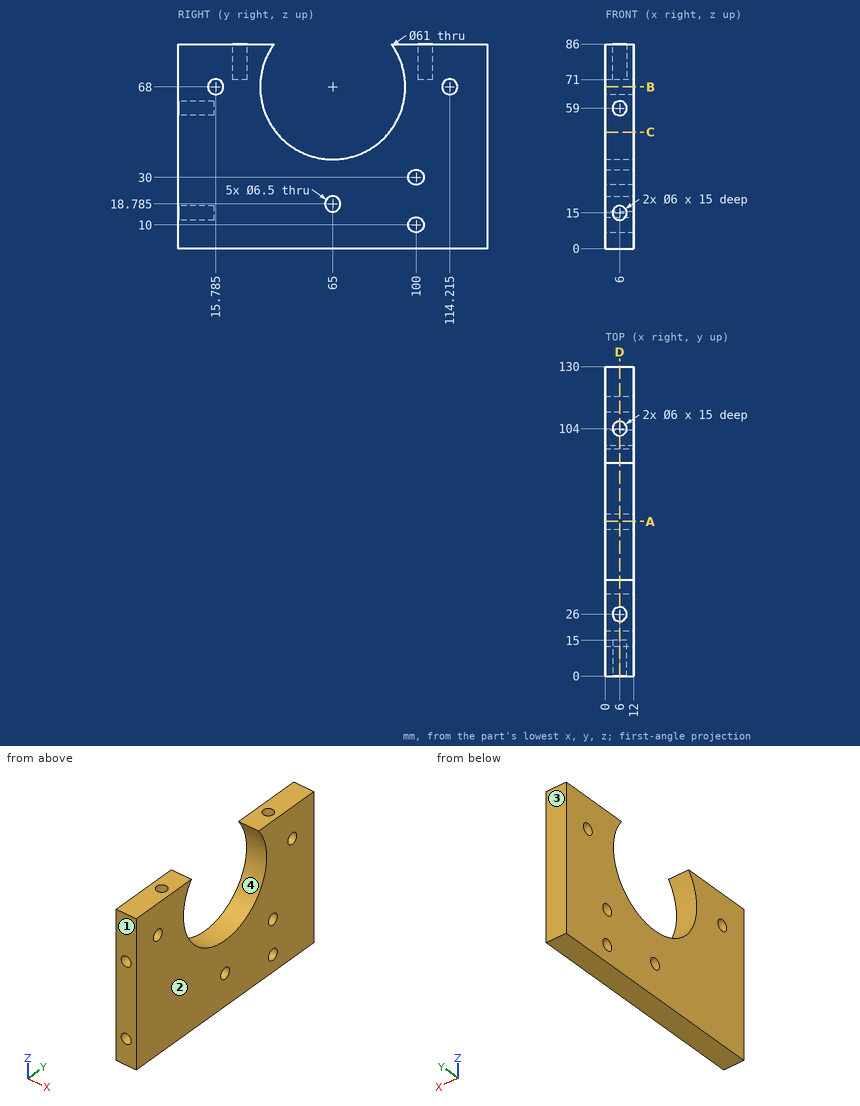
Check sheet for the drawn part. Datum: minimum x, y, z corner. Units: mm. Coordinates: 2 decimals unless noted, no trailing zeros. Order: outer loops, then holes, each group sorted by start corner. A loop starts at its lowest first (then second) coordinate and runs counter-clockwise, first axis right, second up. Notation, with made-up numbers: (83.5, 31) - (89.5, 31) arc R19 ccw to (89.5, 57) - close; hole circle Ø9 at (-34, -4.75). An arc over 180 degrees is marked (long way). Return JSON: item names as keys, results as strings.
(1) Thickness scan on line 1 along Y through (x, z) = (6.25, 68) (1 decimal); line 2 along Z through (x, y) = (6, 9.75); line 3 along Y through (x, z) = (6, 77.75). Record the ranges inside material, lowest first.
Filled sheet:
{"line 1": "y = 0 to 12.5, 19 to 34.5, 95.5 to 111, 117.5 to 130", "line 2": "z = 0 to 12, 18 to 56, 62 to 86", "line 3": "y = 0 to 23, 29 to 36.1, 93.9 to 101, 107 to 130"}
(2) Section check C-C, the plane z = 49. Record the cut outline in (x, y).
Filled sheet:
{"outline": "(0, 0) - (12, 0) - (12, 41.14) - (0, 41.14) - close; (0, 88.86) - (12, 88.86) - (12, 130) - (0, 130) - close"}
(3) Mould release check, pull along Y, two halves, no side actions. Record for the marked faces 1, 2, 3 and 4: pulls with the +Y half, pulls with the -Y half, needs draft (parallel to the pull), parting line crosses it, or undercut.
Filled sheet:
{"face 1": "pulls with the -Y half", "face 2": "needs draft", "face 3": "pulls with the +Y half", "face 4": "undercut"}
(4) Section check D-D, the plane x = 6. Give the number of separate pieces and of enclosed holes in the cut face, and give its area (3 significant figures).
Filled sheet:
{"separate pieces": "1", "enclosed holes": "5", "area": "8,160 mm^2"}
(5) Section check B-B, the plane z = 68. Record the cut outline in (x, y) (1 decimal).
Filled sheet:
{"outline": "(0, 0) - (12, 0) - (12, 12.5) - (0, 12.5) - close; (0, 19) - (12, 19) - (12, 34.5) - (0, 34.5) - close; (0, 95.5) - (12, 95.5) - (12, 111) - (0, 111) - close; (0, 117.5) - (12, 117.5) - (12, 130) - (0, 130) - close"}
(6) Go/stop test with flat-tipped pins: pin 1 (5 mm diameter, centred on x = 5, y = 103.5, fed in from +Z); pin 2 (3 mm diameter, centred on x = 2, y = 75.5, fed in from +Z); pin 3 (1.8 mm diameter, centred on x = 5, z = 16.5, fed in from -Y); pin 4 (6 mm diameter, centred on y = 15.79, z = 68, fed in from -X). Record where each tip stops, or that it passes through.
Filled sheet:
{"pin 1": "stops at z = 86", "pin 2": "stops at z = 39.96", "pin 3": "stops at y = 15", "pin 4": "passes through"}
(7) Section check A-A, the plane y = 65. Record the cut outline in (x, z) (1 decimal).
Filled sheet:
{"outline": "(0, 0) - (12, 0) - (12, 15.5) - (0, 15.5) - close; (0, 22) - (12, 22) - (12, 37.5) - (0, 37.5) - close"}
